```python
from build123d import *

# Parameters (mm, degrees)
F0_R     = 1.5
F1_DEPTH = 15
F2_R     = 1
F3_DEPTH = 10


with BuildPart() as f1:
    # F0 (on Front) → F1 (new body)
    with BuildSketch(Plane.XZ):
        with BuildLine():
            ThreePointArc((-0.5, -5), (-1.9644660941, -1.4644660941), (-5.5, 0))
            ThreePointArc((-5.5, 0), (-9.0355339059, -1.4644660941), (-10.5, -5))
            ThreePointArc((-10.5, -5), (-9.0355339059, -8.5355339059), (-5.5, -10))
            ThreePointArc((-5.5, -10), (-1.9644660941, -8.5355339059), (-0.5, -5))
        make_face()
        with Locations((-5.5, -5)):
            Circle(F0_R, mode=Mode.SUBTRACT)
        with BuildLine():
            Line((5.5, 0), (-5.5, 0))
            ThreePointArc((-5.5, 0), (-1.9644660941, -1.4644660941), (-0.5, -5))
            ThreePointArc((-0.5, -5), (-1.9644660941, -8.5355339059), (-5.5, -10))
            Line((-5.5, -10), (5.5, -10))
            ThreePointArc((5.5, -10), (0.5, -5), (5.5, 0))
        make_face()
        with BuildLine():
            ThreePointArc((10.5, -5), (9.0355339059, -1.4644660941), (5.5, 0))
            ThreePointArc((5.5, 0), (0.5, -5), (5.5, -10))
            ThreePointArc((5.5, -10), (9.0355339059, -8.5355339059), (10.5, -5))
        make_face()
        with Locations((5.5, -5)):
            Circle(F0_R, mode=Mode.SUBTRACT)
    extrude(amount=F1_DEPTH)

    # F2 (on Top) → F3 (cut)
    with BuildSketch(Plane.XY):
        with Locations((0, -10)):
            Circle(F2_R)
    extrude(amount=-F3_DEPTH, mode=Mode.SUBTRACT)


solid = f1.part
```
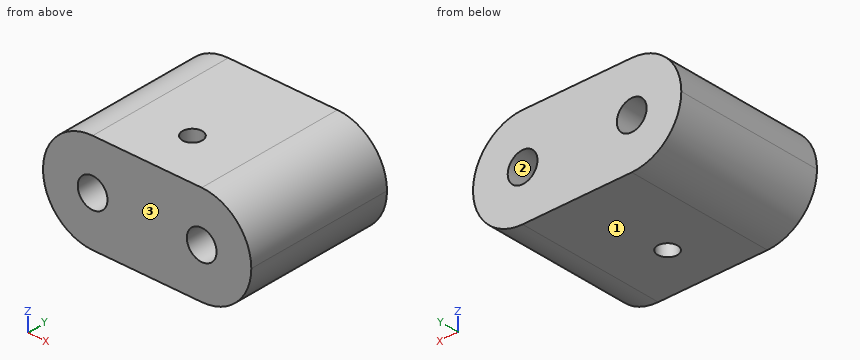
Input: part model. Units: mm. Frame: model coordinates. Face numbers are marked on the shaded views. Round coordinates to 2 decimals unless told otherwise and drop trailing zeros. Loops run counter-clockwise (first coordinate to the right, second up) from the corner with the lowest first, then second, coordinate; pieces in that order, holes last. Notation, with made-up numbers: (28, -19) - (80, -19) arc R21 cw to (80, -12) - close; hole circle Ø1 at (66.5, -13). An arc over 180 degrees is marked (long way). One line per item, written item: value. Start each with the question number.
(1) Section A-A, the plane x = 0. Return loops of the section in (y, z), plus the area to 3 significant figures.
(2) Contact query for flat-ended pins moving along their axis: P1, Ø2.5, axis at x = 5.5, z = -5, coming from the -Y side; P2, Ø2, axis at x = -7.5, y = -6, coming from the +Z side. Output: stop coordinate, or through.
(3) Section D-D, the plane y = -8.5. Return loops of the section in (x, z), plus the area to 3 significant figures.
(4) Section C-C, the plane z = -4.5. Return loops of the section in (x, y), plus the area to 3 significant figures.
(5) Ray query, line 1 (Y direction, x = 0, z = -7); line 2 (Z direction, x = -5.5, y = -9.75); line 3 (X direction, y = -4.5, z = -3.75). Return the intervals inside material, ascending. Write a range as [from, to].
(6) Section B-B, the plane y = -10. Return loops of the section in (x, z).
(7) Draft query along Z for the marked faces 1, 2 and 3. Return one class per face: +Z half, -Z half, draft (parallel to the pull), parting line (faces both ways), or undercut.
Results below:
1. outline: (-15, -10) - (-11, -10) - (-11, 0) - (-15, 0) - close; (-9, -10) - (0, -10) - (0, 0) - (-9, 0) - close
1. area: 130 mm^2
2. P1: through
2. P2: z = -0.1
3. outline: (-5.5, -10) - (5.5, -10) arc R5 ccw to (5.5, 0) - (-5.5, 0) arc R5 ccw to start; hole circle Ø3 at (-5.5, -5); hole circle Ø3 at (5.5, -5)
3. area: 174 mm^2
4. outline: (-10.47, -15) - (-6.91, -15) - (-6.91, 0) - (-10.47, 0) - close; (-4.09, -15) - (4.09, -15) - (4.09, 0) - (-4.09, 0) - close; (6.91, -15) - (10.47, -15) - (10.47, 0) - (6.91, 0) - close; hole circle Ø2 at (0, -10)
4. area: 226 mm^2
5. line 1: [-15, -11], [-9, 0]
5. line 2: [-10, -6.5], [-3.5, 0]
5. line 3: [-10.34, -6.33], [-4.67, 4.67], [6.33, 10.34]
6. outline: (-5.5, -10) - (-1, -10) - (-1, 0) - (-5.5, 0) arc R5 ccw to start; (1, -10) - (5.5, -10) arc R5 ccw to (5.5, 0) - (1, 0) - close; hole circle Ø3 at (-5.5, -5); hole circle Ø3 at (5.5, -5)
7. face 1: -Z half
7. face 2: undercut
7. face 3: draft
